For this review, take the finished solid that the model builds, in its own axes (mm). A direction names the side the tool comes from. Give positions to 0.01 mm unless a question says otherwise; leave off trailing zeros. Loops run counter-clockwise (first coordinate to the right, second up) from the corner with the lowest first, then second, coordinate; pieces in that order, holes last. Notation, with made-up numbers: (-8, 7) -> (13, 7) arc R21 ccw to (13, 23) -> close; hole circle Ø3 at (28.5, 41). An arc over 180 degrees is marked (long way). One line per question, with ' | ' between items. Start each with the question number.
(1) Wall thickness on probe 1 along X at (y, z) = (-3.5, 7.5); probe 2 along X at (y, z) = (7.5, 3.25); probe 3 along X at (y, z) = (12.25, 4): over which ranges is each line inside the solid? List them lowest first.
(2) Tool access review of faces 1 (the flat face through (-15.062, 2.035, 9.343)), 2 (the flat face through (-27.68, 1.66, 7.48)), 3 (the flat face through (-33, 11, 2)), 4 (the flat face through (-24.72, 2.24, 5.91)): name each direction out of +Z, -Z, +X, -X, +Y, -Y from which nothing blocks a thin tool from reaching the whole face with its end or side.
(3) Insertion check: P1, Ø3.5, axis at x = 4.5, y = 10, coming from the +Z side; P2, Ø2.5, axis at x = 3.75, y = 6.27, coming from the -Z side; P3, Ø4, axis at x = -20.5, z = 5, coming from the -Y side; P4, Ø0.9, axis at y = 11.5, z = 3.5, coming from the +X side. Each pin has a flat end and moves straight along its axis. Give the tip position at first contact, or say it passes through.
(4) Consider section B-B (z = 7.25). Give the number of separate pieces and of enclosed holes in the cut face, and give its area (3 significant figures).
(5) Consider section A-A (x = -19). Write out the cut boundary in (y, z), and give its area (3 significant figures).
(6) Draft analysis for pull direction X (two halves, no side actions). For faces 5 (the flat face through (-31, 10.023, 3)), 6 (the flat face through (-29.5, 12, 3)), 7 (the flat face through (-1.819, 0.483, 10.724)), state which applies: +X half, -X half, draft (parallel to the pull), parting line (faces both ways), or undercut.
from build123d import *
from build123d.topology import SkipClean

# Parameters (mm, degrees)
SKETCH2_R           = 1.6
SKETCH2_W           = 28.5
SKETCH2_H           = 12
BOSS_EXTRUDE1_DEPTH = 2
SKETCH3_W           = 44.5
SKETCH3_H           = 15
BOSS_EXTRUDE2_DEPTH = 7
BOSS_EXTRUDE3_REACH = 44.543
SKETCH2_3_R         = 1.6
SKETCH2_3_W         = 28.5
SKETCH2_3_H         = 12
SKETCH4_R           = 2.010738951
SKETCH4_R_2         = 2
CUT_EXTRUDE1_DEPTH  = 2
SKETCH4_2_R         = 2
SKETCH4_2_R_2       = 2.010738951
CUT_EXTRUDE2_DEPTH  = 42.581180746
BOSS_EXTRUDE4_DEPTH = 44.5


with BuildPart() as part:
    # Sketch2 → Boss-Extrude1 (new body)
    # profile 1 of 6: a face of its own
    with BuildSketch(Plane.XY):
        with BuildLine():
            ThreePointArc((3.38, 10.004825556), (6.267439172, 9.052511956), (7.5, 6.27312354))
            Line((7.5, 6.27312354), (7.5, 13))
            Line((7.5, 13), (0, 13))
            Line((0, 13), (0, 10.023123532))
            Line((0, 10.023123532), (3.38, 10.023123532))
            Line((3.38, 10.023123532), (3.38, 10.004825556))
        make_face()
    # profile 2 of 6: a face of its own
    with BuildSketch(Plane.XY):
        with BuildLine():
            Line((3.38, 2.523123532), (0, 2.523123532))
            Line((0, 2.523123532), (0, 0))
            Line((0, 0), (7.5, 0))
            Line((7.5, 0), (7.5, 6.27312354))
            ThreePointArc((7.5, 6.27312354), (6.401650432, 3.621473105), (3.75, 2.523123532))
            Line((3.75, 2.523123532), (3.725156678, 2.523123532))
            Line((3.725156678, 2.523123532), (3.38, 2.523123532))
        make_face()
    # profile 3 of 6: a face of its own
    with BuildSketch(Plane.XY):
        with BuildLine():
            Line((-37, 13), (-37, 6.643123532))
            ThreePointArc((-37, 6.643123532), (-35.64002092, 9.18640347), (-32.88, 10.023123532))
            Line((-32.88, 10.023123532), (-29.5, 10.023123532))
            Line((-29.5, 10.023123532), (-29.5, 13))
            Line((-29.5, 13), (-37, 13))
        make_face()
    # profile 4 of 6: a face of its own
    with BuildSketch(Plane.XY):
        with BuildLine():
            Line((-37, 0), (-29.5, 0))
            Line((-29.5, 0), (-29.5, 2.523123532))
            Line((-29.5, 2.523123532), (-32.88, 2.523123532))
            ThreePointArc((-32.88, 2.523123532), (-35.64002092, 3.359843593), (-37, 5.903123532))
            Line((-37, 5.903123532), (-37, 0))
        make_face()
    # profile 5 of 6: a face of its own
    with BuildSketch(Plane.XY):
        with BuildLine():
            Line((3.38, 10.004825556), (0, 10.023123532))
            Line((0, 10.023123532), (0, 13))
            Line((0, 13), (-29.5, 13))
            Line((-29.5, 13), (-29.5, 10.023123532))
            Line((-29.5, 10.023123532), (-32.88, 10.023123532))
            Line((-32.88, 10.023123532), (-32.88, 10.004825556))
            ThreePointArc((-32.88, 10.004825556), (-37, 6.273123532), (-32.88, 2.541421507))
            Line((-32.88, 2.541421507), (-32.88, 2.523123532))
            Line((-32.88, 2.523123532), (-29.5, 2.523123532))
            Line((-29.5, 2.523123532), (-29.5, 0))
            Line((-29.5, 0), (0, 0))
            Line((0, 0), (0, 2.523123532))
            Line((0, 2.523123532), (3.38, 2.523123532))
            Line((3.38, 2.523123532), (3.38, 2.541421507))
            ThreePointArc((3.38, 2.541421507), (7.5, 6.273123532), (3.38, 10.004825556))
        make_face()
        with Locations((3.75, 6.273123532)):
            Circle(SKETCH2_R, mode=Mode.SUBTRACT)
        with Locations((-33.25, 6.273123532)):
            Circle(SKETCH2_R, mode=Mode.SUBTRACT)
        with Locations((-14.75, 6.5)):
            Rectangle(SKETCH2_W, SKETCH2_H, mode=Mode.SUBTRACT)
    # profile 6 of 6: a face of its own
    with BuildSketch(Plane.XY):
        with Locations((-14.75, 6.5)):
            Rectangle(SKETCH2_W, SKETCH2_H)
    extrude(amount=BOSS_EXTRUDE1_DEPTH)

    # Sketch3 → Boss-Extrude2 (add)
    with BuildSketch(Plane(origin=(0, -1.778051923, -0.647157975), x_dir=(1, 0, 0), z_dir=(-1.5523980964466968e-15, 0.9396926207859094, 0.34202014332566594))):
        with Locations((-14.75, -8.188691132)):
            Rectangle(SKETCH3_W, SKETCH3_H)
    extrude(amount=BOSS_EXTRUDE2_DEPTH)

    # Boss-Extrude3: up to this plane
    with SkipClean():  # the faces are left unmerged after this step: merging them gives an invalid solid
        boss_extrude3_end = Plane(origin=(-37, 4.564250183, 2.394141003), z_dir=(0, -0.34202014332566594, 0.9396926207859094))
        # Sketch2<3> → Boss-Extrude3 (add, up to the surface)
        with BuildSketch(Plane.XY, mode=Mode.PRIVATE) as boss_extrude3_sk1:
            with BuildLine():
                Line((3.38, 10.004825556), (0, 10.023123532))
                Line((0, 10.023123532), (0, 13))
                Line((0, 13), (-29.5, 13))
                Line((-29.5, 13), (-29.5, 10.023123532))
                Line((-29.5, 10.023123532), (-32.88, 10.023123532))
                Line((-32.88, 10.023123532), (-32.88, 10.004825556))
                ThreePointArc((-32.88, 10.004825556), (-37, 6.273123532), (-32.88, 2.541421507))
                Line((-32.88, 2.541421507), (-32.88, 2.523123532))
                Line((-32.88, 2.523123532), (-29.5, 2.523123532))
                Line((-29.5, 2.523123532), (-29.5, 0))
                Line((-29.5, 0), (0, 0))
                Line((0, 0), (0, 2.523123532))
                Line((0, 2.523123532), (3.38, 2.523123532))
                Line((3.38, 2.523123532), (3.38, 2.541421507))
                ThreePointArc((3.38, 2.541421507), (7.5, 6.273123532), (3.38, 10.004825556))
            make_face()
            with Locations(Location((3.75, 6.273123532, 0), (0, 0, 270))):
                Circle(SKETCH2_3_R, mode=Mode.SUBTRACT)
            with Locations(Location((-33.25, 6.273123532, 0), (0, 0, 270))):
                Circle(SKETCH2_3_R, mode=Mode.SUBTRACT)
            with Locations((-14.75, 6.5)):
                Rectangle(SKETCH2_3_W, SKETCH2_3_H, mode=Mode.SUBTRACT)
        boss_extrude3_tool1 = split(extrude(boss_extrude3_sk1.sketch, amount=BOSS_EXTRUDE3_REACH, mode=Mode.PRIVATE), bisect_by=boss_extrude3_end, keep=Keep.BOTH, mode=Mode.PRIVATE)
        add(boss_extrude3_tool1.solids().sort_by_distance((1.68749, 9.550381, 0))[0])
        # Sketch2<3> → Boss-Extrude3 (add, up to the surface)
        with BuildSketch(Plane.XY, mode=Mode.PRIVATE) as boss_extrude3_sk2:
            with Locations((-14.75, 6.5)):
                Rectangle(SKETCH2_3_W, SKETCH2_3_H)
        boss_extrude3_tool2 = split(extrude(boss_extrude3_sk2.sketch, amount=BOSS_EXTRUDE3_REACH, mode=Mode.PRIVATE), bisect_by=boss_extrude3_end, keep=Keep.BOTH, mode=Mode.PRIVATE)
        add(boss_extrude3_tool2.solids().sort_by_distance((-14.75, 6.5, 0))[0])

    # Sketch4 → Cut-Extrude1 (cut)
    # profile 1 of 2: a face of its own
    with SkipClean():  # the faces are left unmerged after this step: merging them gives an invalid solid
        with BuildSketch(Plane(origin=(0, 4.799796423, 1.746983028), x_dir=(1, 0, 0), z_dir=(-1.5524032942846936e-15, 0.9396926207859094, 0.34202014332566594))):
            Polygon((-28.67598183, -8.188691132), (-26.712990915, -11.588691132), (-22.787009085, -11.588691132), (-20.82401817, -8.188691132), (-22.787009085, -4.788691132), (-26.712990915, -4.788691132), align=None)
            with Locations(Location((-24.75, -8.188691132, 0), (0, 0, 270))):
                Circle(SKETCH4_R, mode=Mode.SUBTRACT)
        # profile 2 of 2: a face of its own
        with BuildSketch(Plane(origin=(0, 4.799796423, 1.746983028), x_dir=(1, 0, 0), z_dir=(-1.5524032942846936e-15, 0.9396926207859094, 0.34202014332566594))):
            Polygon((-8.67598183, -8.188691132), (-6.712990915, -11.588691132), (-2.787009085, -11.588691132), (-0.82401817, -8.188691132), (-2.787009085, -4.788691132), (-6.712990915, -4.788691132), align=None)
            with Locations(Location((-4.75, -8.188691132, 0), (0, 0, 270))):
                Circle(SKETCH4_R_2, mode=Mode.SUBTRACT)
        extrude(amount=-CUT_EXTRUDE1_DEPTH, mode=Mode.SUBTRACT)

    # Sketch4<2> → Cut-Extrude2 (cut, through all)
    with SkipClean():  # the faces are left unmerged after this step: merging them gives an invalid solid
        with BuildSketch(Plane(origin=(0, 4.799796423, 1.746983028), x_dir=(1, 0, 0), z_dir=(-1.5524032942846936e-15, 0.9396926207859094, 0.34202014332566594))):
            with Locations(Location((-4.75, -8.188691132, 0), (0, 0, 270))):
                Circle(SKETCH4_2_R)
            with Locations(Location((-24.75, -8.188691132, 0), (0, 0, 270))):
                Circle(SKETCH4_2_R_2)
        extrude(amount=-CUT_EXTRUDE2_DEPTH, mode=Mode.SUBTRACT)

    # Sketch5 → Boss-Extrude4 (add)
    with SkipClean():  # the faces are left unmerged after this step: merging them gives an invalid solid
        with BuildSketch(Plane(origin=(7.5, 0, 0), x_dir=(0, 0, -1), z_dir=(1, 0, 0))):
            Polygon((-0.732889795, 0), (0, 0), (0, -2.013598163), align=None)
        extrude(amount=-BOSS_EXTRUDE4_DEPTH)


solid = part.part
A:
1) probe 1: x = -37 to -26.76, -22.74 to -6.75, -2.75 to 7.5 | probe 2: x = -36.79 to -34.28, -32.22 to 2.72, 4.78 to 7.29 | probe 3: x = -29.5 to 0
2) face 1: +Z, +X, -X | face 2: none | face 3: +Z, -X, +Y | face 4: +Z
3) P1: stops at z = 4.38 | P2: passes through | P3: stops at y = -4.56 | P4: stops at x = 0
4) separate pieces: 3 | enclosed holes: 0 | area: 270 mm^2
5) outline: (-7.14, 14.1) -> (-2.01, 0) -> (13, 0) -> (13, 5.46) -> (4.56, 2.39) -> (-0.57, 16.49) -> close | area: 146 mm^2
6) face 5: draft | face 6: -X half | face 7: undercut
